For this review, take the finished solid that the model builds, in its own axes (mm). Face numbers are marked on the shaded views. A direction names the side the tool comes from. Give positions to 0.01 mm unless a question says otherwise; leave off trailing zeros. Write each loop counter-clockwise with the first axis right and the second up, starting at its lowest first coordinate (ties: lowest second). Pieces come first, ordered by that corner, then holes. Notation, with made-up numbers: M -2,25 L 10,25 A16 ccw 10,47 Z; hole C 50.25,2.25 d10. An arc over 180 degrees is marked long. Use one line per item in the form item = value. Start each with the question number.
Q1. Consider section D-D on z = -105. Write out the cut boundary in (x, y).
Q2. For probe 1 along Z at (x, y) = (69, -7.5); probe 2 along Z at (x, y) = (589, -381.5); probe 3 along Y at (x, z) = (101, 49.5), list the stretches that pass through material, from the lowest coordinate up. Write a range as [from, to].
Q3. Consider section A-A on x = 346. Write out the cut boundary in (y, z), and give its area (3 significant figures).
Q4. Clearance check with flat-ended pins moving along their axes: pin 1 Ø19 at (y, z) = (-430.5, -7) entering from -X; pin 2 Ø5 at (x, y) = (161, 310.5) entering from +Z; pin 3 Ø12 at (x, y) = (-367, -367) entering from -Z. State where each tip first meets the part, or that it passes through.
Q5. Mouldability with a two-part tool opening along X and no side actions: class the marked faces 3 and 4 as released by +X, released by -X, zero draft, split by the parting line, or undercut.
Q6. Consider section B-B on z = 74. Write out the cut boundary in (x, y).
Q7. Consider section C-C on y = -120. Write out the cut boundary in (x, z).
Q8. Tool access review of the marked faces 1 and 2: name each direction out of +Z, -Z, +X, -X, +Y, -Y from which nothing blocks a thin tool from reaching the whole face with its end or side.
```python
from build123d import *

# Parameters (mm, degrees)
SKETCH1_W           = 1384.3
SKETCH1_H           = 838.2
BOSS_EXTRUDE1_DEPTH = 25.4
CHAMFER1_SIZE       = 10
SKETCH2_W           = 1333.5
SKETCH2_H           = 749.3
CUT_EXTRUDE1_DEPTH  = 6.35
SKETCH3_W           = 533.4
SKETCH3_H           = 330.2
BOSS_EXTRUDE2_DEPTH = 38.1
CHAMFER2_SIZE       = 20


with BuildPart() as part:
    # Sketch1 → Boss-Extrude1 (new body)
    with BuildSketch(Plane.XY):
        Rectangle(SKETCH1_W, SKETCH1_H)
    extrude(amount=BOSS_EXTRUDE1_DEPTH)

    # Chamfer1
    chamfer1_edges = [part.edges().sort_by_distance(p)[0] for p in [
        (-692.15, 0, 25.4),
        (692.15, 0, 25.4),
        (0, 419.1, 25.4),
    ]]
    chamfer(chamfer1_edges, length=CHAMFER1_SIZE)

    # Sketch2 → Cut-Extrude1 (cut)
    with BuildSketch(Plane.XY.offset(25.4)):
        Rectangle(SKETCH2_W, SKETCH2_H)
    extrude(amount=-CUT_EXTRUDE1_DEPTH, mode=Mode.SUBTRACT)

    # Sketch3 → Boss-Extrude2 (add)
    with BuildSketch(Plane.XZ.offset(419.1)):
        with Locations((0, 12.7)):
            Rectangle(SKETCH3_W, SKETCH3_H)
    extrude(amount=BOSS_EXTRUDE2_DEPTH)

    # Chamfer2
    chamfer2_edges = [part.edges().sort_by_distance(p)[0] for p in [
        (266.7, -419.1, 101.6),
        (-266.7, -419.1, 101.6),
        (0, -419.1, 177.8),
    ]]
    chamfer(chamfer2_edges, length=CHAMFER2_SIZE)


solid = part.part
```
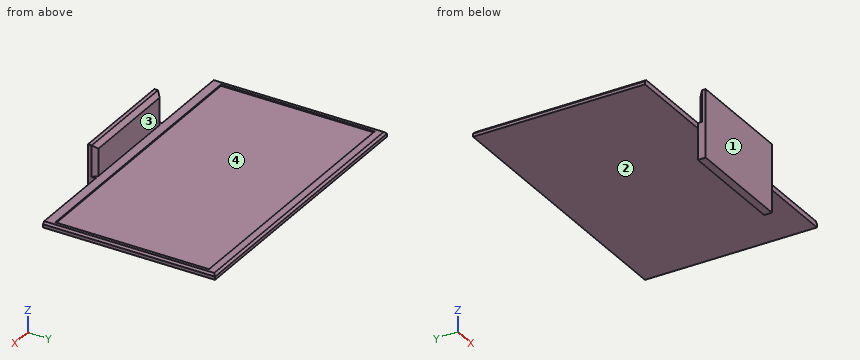
Working result:
q1.outline = M -266.7,-457.2 L 266.7,-457.2 L 266.7,-419.1 L -266.7,-419.1 Z
q2.probe_1 = [0, 19.05]
q2.probe_2 = [0, 25.4]
q2.probe_3 = [-457.2, -419.1]
q3.outline = M -419.1,0 L 419.1,0 L 419.1,15.4 L 409.1,25.4 L 374.65,25.4 L 374.65,19.05 L -374.65,19.05 L -374.65,25.4 L -419.1,25.4 Z
q3.area = 16,500 mm²
q4.pin_1 = -266.7
q4.pin_2 = 19.05
q4.pin_3 = 0
q5.face_3 = zero draft
q5.face_4 = undercut
q6.outline = M -266.7,-457.2 L 266.7,-457.2 L 266.7,-439.1 L 246.7,-419.1 L -246.7,-419.1 L -266.7,-439.1 Z
q7.outline = M -692.15,0 L 692.15,0 L 692.15,15.4 L 682.15,25.4 L 666.75,25.4 L 666.75,19.05 L -666.75,19.05 L -666.75,25.4 L -682.15,25.4 L -692.15,15.4 Z
q8.face_1 = +Z, -Z, +X, -X, -Y
q8.face_2 = -Z, +X, -X, +Y
